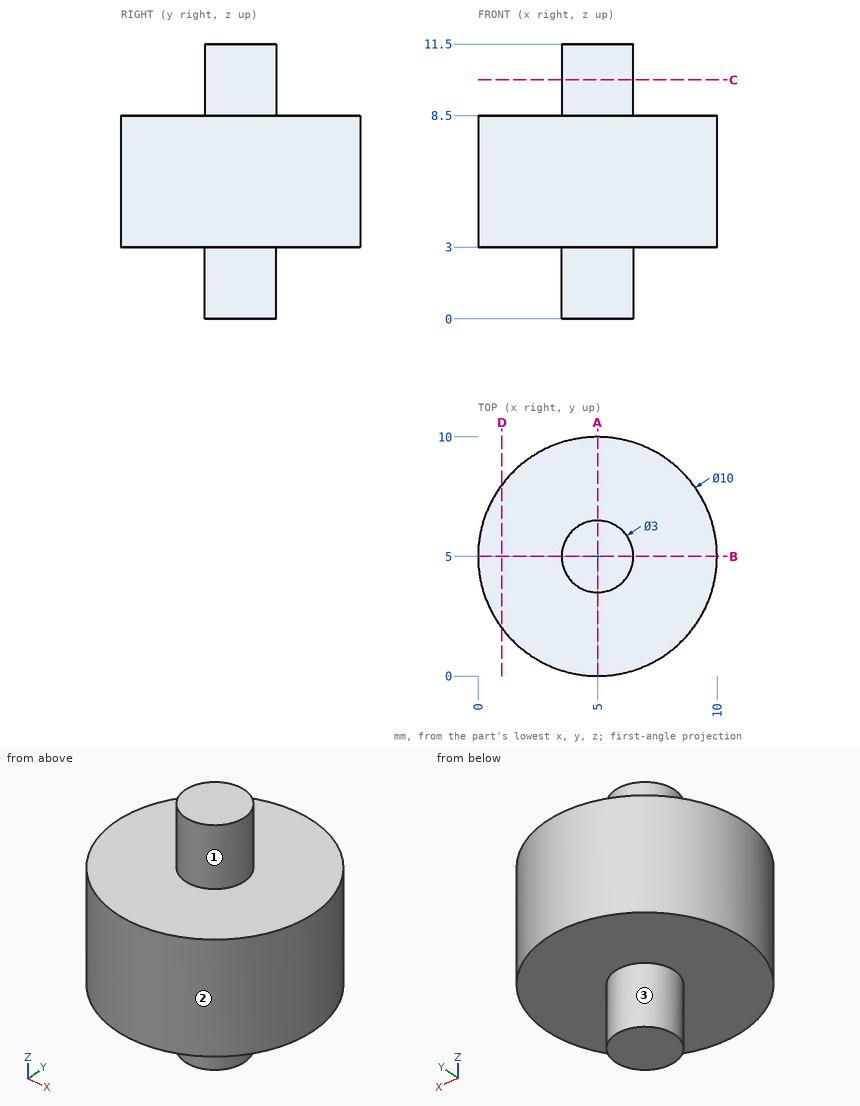
Here's the drawing with two shaded views (mm, measured from the low corner). I have some questions. A direction names the side the tool comes from. Coordinates: 2 decimals unless noted, no trailing zeros. Write each loop counter-clockwise with the first axis right and the second up, starting at its lowest first coordinate (ties: lowest second). Pieces come first, ordered by that corner, then holes.
Item 1: I want a section at A-A on x = 5. Write out the boundary of the cut face in (y, z), and give its area (3 significant figures).
Item 2: On a 3-axis mill with a long thin cutter (end or side, diameter ignored), from which of +Z, -Z, +X, -X, +Y, -Y can I reach the whole of each face in a straight line? I mean the marked faces 1, 2 and 3. Say none if no direction works.
Item 3: I want a section at D-D on x = 1. Write out the boundary of the cut face in (y, z).
Item 4: Will these pins go through, and if not, where does the flat tip stop? pin 1 (3 mm diameter, centred on x = 4.5, y = 5.5, fed in from -Z); pin 2 (2 mm diameter, centred on x = 2.5, y = 9, fed in from -Z); pin 3 (5 mm diameter, centred on x = 1.5, z = 7.5, fed in from +Y).
Item 5: If I drill on line 1 (Z direction, x = 4.75, y = 8.5); line 2 (X direction, y = 8, z = 4); line 3 (X direction, y = 0.5, z = 6.5), over which ranges is the centre line in solid material (lowest first)?
Item 6: I want a section at C-C on z = 10. Write out the boundary of the cut face in (x, y).
Findings below:
1. outline: (0, 3) - (3.5, 3) - (3.5, 0) - (6.5, 0) - (6.5, 3) - (10, 3) - (10, 8.5) - (6.5, 8.5) - (6.5, 11.5) - (3.5, 11.5) - (3.5, 8.5) - (0, 8.5) - close
1. area: 73.0 mm2
2. face 1: +Z
2. face 2: +Z, -Z
2. face 3: -Z
3. outline: (2, 3) - (8, 3) - (8, 8.5) - (2, 8.5) - close
4. pin 1: stops at z = 0
4. pin 2: stops at z = 3
4. pin 3: stops at y = 9.9
5. line 1: z = 3 to 8.5
5. line 2: x = 1 to 9
5. line 3: x = 2.82 to 7.18
6. outline: circle Ø3 at (5, 5)
